Print and shaded views of the part. All mm, measured from the part's lowest x, y and z. A direction names the side the tool comes from. Round coordinates to 2 decimals unless told otherwise and drop trailing zeros. Write each loop counter-clockwise with the first axis right and the second up, starting at its lowest first coordinate (ties: lowest second). Pieces come first, ordered by that corner, then holes. Notation, with made-up numbers: M -29.75,53.5 L 13.25,53.5 A7 cw 13.25,59.5 Z; hole C 89,83 d1. An arc over 180 degrees is marked long. Write item = value, one per line. Start each with the question number.
Q1. Tool access for the marked faces 1 and 2: list every direction of +Z, -Z, +X, -X, +Y, -Y with a clear straight run to the whole face (end or side of a thin tool).
Q2. Band-saw the part on A-A on y = 12. Write the cut outline in (x, z) (3 decimals).
Q3. Band-saw the part on C-C on z = 1.5. Write the cut outline in (x, y) (3 decimals), plus the area to 3 significant figures.
Q4. Band-saw the part on D-D on z = 6.75. Write the cut outline in (x, y) (3 decimals), plus the area to 3 significant figures.
Q5. Probe L1, parallel to X at y = 12, z = 5.25 (3 decimals); L2, parallel to Z at x = 1.75, y = 11.75; L3, parallel to X at y = 13, z = 8.5. List the from-to ranges inside material, lowest first.
Q6. Pull direction Z, two halves, no side cores. Call the marked faces 3, 4 and 5: released by +Z, released by -Z, zero draft, split by the parting line, or undercut.
Q7. Drop flat-ended pins along their axis: P1, Ø1, axis at y = 17.5, z = 4, coming from the +X side; P2, Ø4, axis at x = 12, y = 12, coming from the -Z side; P3, Ø4, axis at y = 7, z = 4, coming from the -X side. Give the stop position or say it passes through.
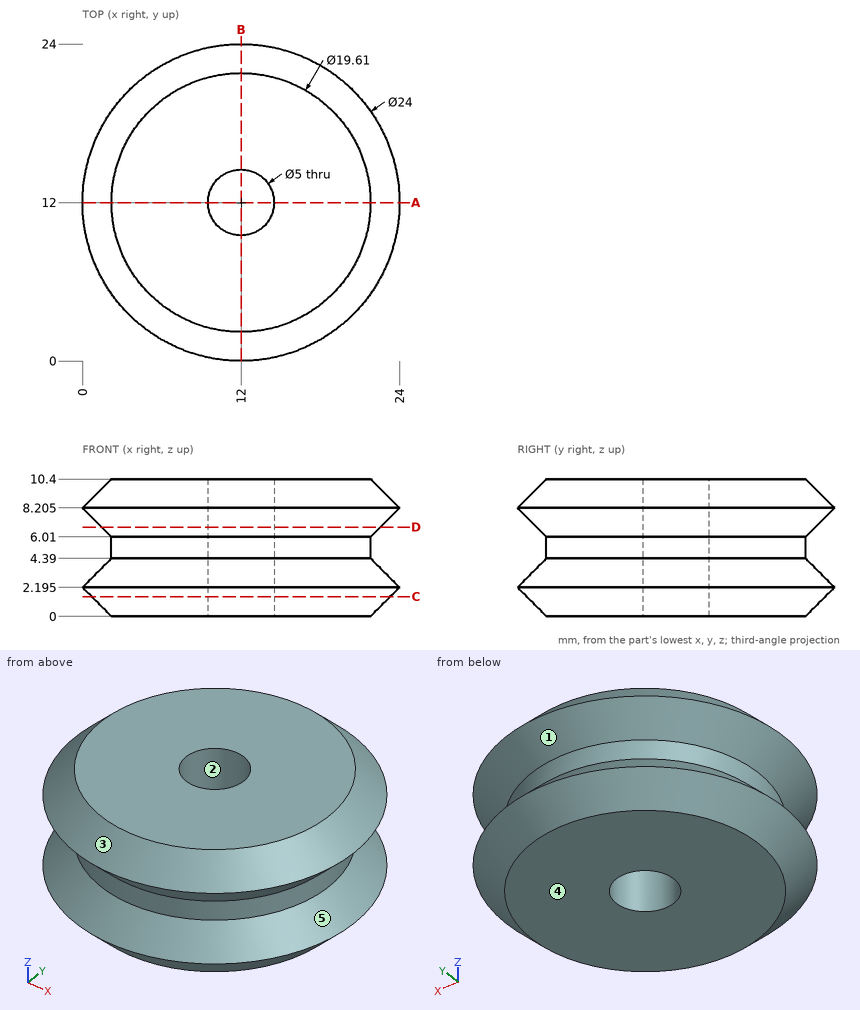
Conclusion:
q1.face_1 = none
q1.face_2 = +Z, -Z
q2.outline = M 0,2.195 L 2.195,0 L 9.5,0 L 9.5,10.4 L 2.195,10.4 L 0,8.205 L 2.195,6.01 L 2.195,4.39 Z; M 14.5,0 L 21.805,0 L 24,2.195 L 21.805,4.39 L 21.805,6.01 L 24,8.205 L 21.805,10.4 L 14.5,10.4 Z
q3.outline = C 12,12 d22.61; hole C 12,12 d5
q3.area = 382 mm^2
q4.outline = C 12,12 d21.09; hole C 12,12 d5
q4.area = 330 mm^2
q5.L1 = 2.195 to 9.5, 14.5 to 21.805
q5.L2 = 0.45 to 3.94, 6.46 to 9.95
q5.L3 = 0.34 to 9.71, 14.29 to 23.66
q6.face_3 = released by +Z
q6.face_4 = released by -Z
q6.face_5 = undercut
q7.P1 = 21.24
q7.P2 = through
q7.P3 = 0.74
